Part model, mm, in its own coordinate system. Face numbers are marked on the shaded views. A direction names the side the tool comes from. Coordinates: 2 decimals unless noted, no trailing zeros. Write each loop counter-clockwise with the first axis right and the second up, starting at its lowest first coordinate (ties: lowest second). Pieces come first, ordered by that corner, then holes. Notation, with made-up numbers: (7, -20) -> (29, -20) arc R21 ccw to (29, 7) -> close; hole circle Ø6 at (-19.5, 68.5). An arc over 180 degrees is marked (long way). One line per question, with ' | ' between items. Start each with the question number.
Item 1: Saw through at A-A (z = -40.5). List the corners of the cut face in (x, y) (3 decimals).
Item 2: Saw through at D-D (z = -14). List the corners of the cut face in (x, y).
Item 3: Saw through at B-B (x = 28). List the corners of the cut face in (y, z), and give its area (3 significant figures).
Item 4: Pin check, flat tips, straight feed: pin 1 (0.8 mm diameter, centred on x = 74.5, z = 22, fed in from +Y); pin 2 (1.3 mm diameter, centred on y = 28.5, z = 62.5, fed in from -X); pin 3 (12 mm diameter, centred on y = 19, z = -34.5, fed in from -X). Stop position of each tip, or through.
Item 5: Probe probe 1 along Z at (x, y) = (-28.5, 29); probe 2 along Y at (x, z) = (56.5, 32); probe 3 along X at (y, z) = (29, 40). List the from-to ranges inside material, lowest first. Write a range as [from, to].
Item 6: Saw through at C-C (y = 27.94). Count the separate pieces of the cut face and the enclosed holes in it, and give its area (3 significant figures).
Item 7: Two-plate mould, pull along Z, no slides. Class the marked faces 3, 4 and 5: pulls with the +Z half, pulls with the -Z half, needs draft (parallel to the pull), parting line crosses it, or undercut.
Item 8: 3-axis set-ups, long thin cutter, end or side, ignore diameter. For the marked faces 1 and 2: which of +Z, -Z, +X, -X, +Y, -Y reach the whole face in a straight line?
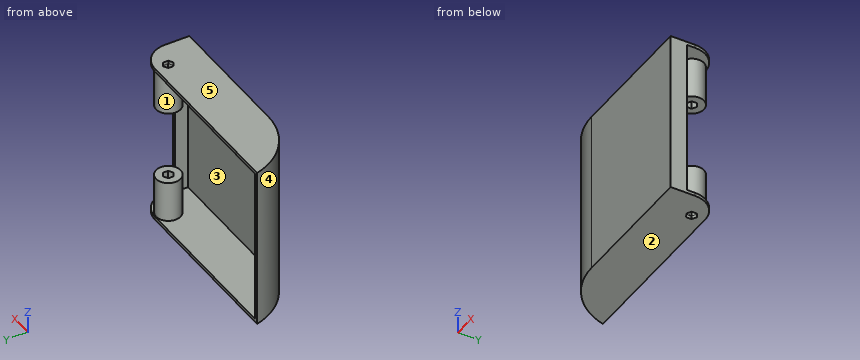
from build123d import *

# Parameters (mm, degrees)
SKETCH1_W               = 152.4
SKETCH1_H               = 127
BOSS_EXTRUDE1_DEPTH     = 38.1
FILLET1_R               = 50.8
SHELL1_T                = -2.54
CUT_EXTRUDE2_DEPTH      = 151.825533647
CUT_EXTRUDE2_DEPTH_BACK = 151.825533647
SKETCH4_R               = 9.525
BOSS_EXTRUDE2_DEPTH     = 124.46
SKETCH2_W               = 11.613456366
SKETCH2_H               = 121.92
CUT_EXTRUDE3_DEPTH      = 25.4
SKETCH5_W               = 29.081811675
SKETCH5_H               = 58.42
CUT_EXTRUDE4_DEPTH      = 50.8
FILLET3_R               = 19.05


with BuildPart() as part:
    # Sketch1 → Boss-Extrude1 (new body)
    with BuildSketch(Plane(origin=(0, 0, 0), x_dir=(1, 0, 0), z_dir=(0, 1, 0))):
        Rectangle(SKETCH1_W, SKETCH1_H)
    extrude(amount=BOSS_EXTRUDE1_DEPTH)

    # Fillet1
    # the kernel refuses this fillet: 50.8 mm, written as the material it takes off along each edge
    with BuildSketch(Plane(origin=(-76.2, 0, -186.467221242), x_dir=(0, 1, 0), z_dir=(0, 0, 1))) as fillet1_piece_1:
        with BuildLine():
            CenterArc((50.8, -49.186888497), FILLET1_R, 104.477512186, 75.522487814)
            Line((0, -49.186888497), (-1.016, -49.186888497))
            Line((-1.016, -49.186888497), (-1.016, 0))
            Line((-1.016, 0), (0, 1.016))
            ThreePointArc((0, 1.016), (19.05, 1.016), (37.846, 0.98373777))
            Line((37.846, 0.98373777), (38.1, 0))
        make_face()
    extrude(amount=372.934442484, mode=Mode.SUBTRACT)

    # Shell1
    shell1_openings = [part.faces().sort_by_distance(p)[0] for p in [
        (0, 38.1, 0),
    ]]
    offset(amount=SHELL1_T, openings=shell1_openings, kind=Kind.INTERSECTION)

    # Sketch3 → Cut-Extrude2 (cut, two sides: drawn at the far end of the back side and taken through both)
    with BuildSketch(Plane.XY.offset(-60.96).offset(-CUT_EXTRUDE2_DEPTH_BACK)):
        Polygon((56.572208389, 32.046115114), (53.016208389, 29.993057557), (53.016208389, 25.886942443), (56.572208389, 23.833884886), (60.128208389, 25.886942443), (60.128208389, 29.993057557), align=None)
    extrude(amount=CUT_EXTRUDE2_DEPTH + CUT_EXTRUDE2_DEPTH_BACK, mode=Mode.SUBTRACT)

    # Sketch4 → Boss-Extrude2 (add)
    with BuildSketch(Plane.XY.offset(-60.96)):
        with Locations(Location((56.706906113, 27.94, 0), (0, 0, 180))):
            Circle(SKETCH4_R)
        Polygon((56.706906113, 32.046115114), (53.150906113, 29.993057557), (53.150906113, 25.886942443), (56.706906113, 23.833884886), (60.262906113, 25.886942443), (60.262906113, 29.993057557), align=None, mode=Mode.SUBTRACT)
    extrude(amount=BOSS_EXTRUDE2_DEPTH)

    # Sketch2 → Cut-Extrude3 (cut)
    with BuildSketch(Plane(origin=(0, 38.1, 0), x_dir=(1, 0, 0), z_dir=(0, 1, 0))):
        with Locations((78.243168089, 0)):
            Rectangle(SKETCH2_W, SKETCH2_H)
    extrude(amount=-CUT_EXTRUDE3_DEPTH, mode=Mode.SUBTRACT)

    # Sketch5 → Cut-Extrude4 (cut)
    with BuildSketch(Plane(origin=(0, 2.54, 0), x_dir=(1, 0, 0), z_dir=(0, 1, 0))):
        with Locations((53.93192453, 0)):
            Rectangle(SKETCH5_W, SKETCH5_H)
    extrude(amount=CUT_EXTRUDE4_DEPTH, mode=Mode.SUBTRACT)

    # Fillet3
    fillet3_edges = [part.edges().sort_by_distance(p)[0] for p in [
        (76.2, 38.1, 62.23),
        (76.2, 38.1, -62.23),
    ]]
    fillet(fillet3_edges, radius=FILLET3_R)


solid = part.part
From the geometry:
1) outline: (-76.2, 38.1) arc R50.8 ccw to (-27.013, 0) -> (76.2, 0) -> (76.2, 12.7) -> (73.66, 12.7) -> (73.66, 2.54) -> (-27.013, 2.54) arc R48.26 cw to (-73.572, 38.1) -> close; circle Ø19.05 at (56.707, 27.94); hole (53.151, 25.887) -> (56.707, 23.834) -> (60.263, 25.887) -> (60.263, 29.993) -> (56.707, 32.046) -> (53.151, 29.993) -> close
2) outline: (-76.2, 38.1) arc R50.8 ccw to (-27.01, 0) -> (76.2, 0) -> (76.2, 12.7) -> (73.66, 12.7) -> (73.66, 2.54) -> (-27.01, 2.54) arc R48.26 cw to (-73.57, 38.1) -> close
3) outline: (0, -63.5) -> (38.1, -63.5) -> (38.1, -60.96) -> (2.54, -60.96) -> (2.54, 60.96) -> (38.1, 60.96) -> (38.1, 63.5) -> (0, 63.5) -> close | area: 503 mm2
4) pin 1: y = 12.7 | pin 2: x = -72.97 | pin 3: x = -70.77
5) probe 1: [-63.5, -60.96], [60.96, 63.5] | probe 2: [0, 2.54], [18.42, 23.95], [31.93, 37.46] | probe 3: [-72.9, -70.07], [47.24, 53.15], [60.26, 66.17]
6) separate pieces: 3 | enclosed holes: 0 | area: 1,810 mm2
7) face 3: undercut | face 4: needs draft | face 5: pulls with the +Z half
8) face 1: none | face 2: -Z, +X, -X, +Y, -Y
